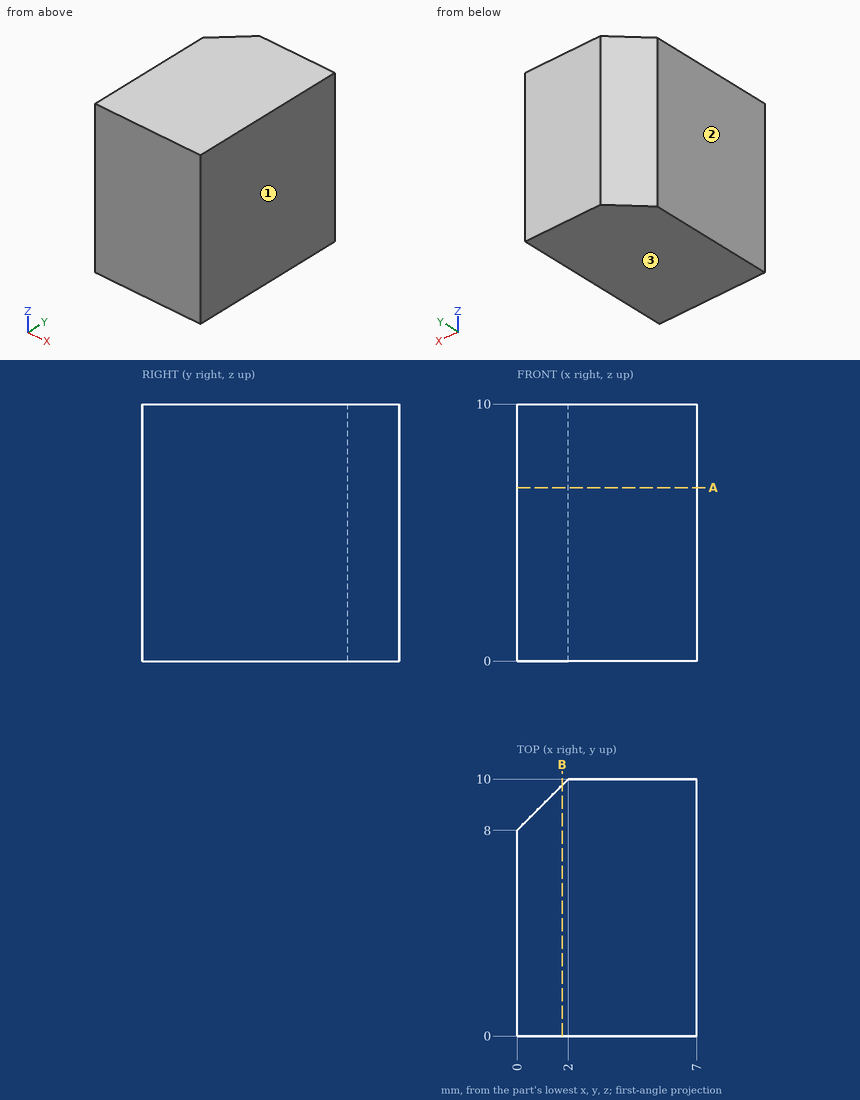
Answer from the drawing. Dimensions are ordinates in mm from the lowest x, y and z of the part. Give positions to 0.01 mm unless a question says otherwise; leave off trailing zeros. Loops run counter-clockwise (first coordinate to the right, second up) from the corner with the lowest first, then second, coordinate; pieces in that order, holes last.
Item 1: Find the intervals of material crossed by line 1 along Y through (x, z) = (0.5, 2.5); line 2 along X through (y, z) = (8.5, 3); line 3 along Y through (x, z) = (1.5, 4.5), in increasing order.
Item 2: The mould has two halves that part along X. Classify the marked faces 1, 2 and 3: released by +X, released by -X, zero draft, split by the parting line, or undercut.
Item 3: The part is cut by section A-A (z = 6.75). Write down the section's boundary in (x, y), and give its area (3 significant figures).
Item 4: The part is cut by section B-B (x = 1.75). Write down the section's boundary in (y, z).
Taken from the geometry:
1. line 1: y = 0 to 8.5
1. line 2: x = 0.5 to 7
1. line 3: y = 0 to 9.5
2. face 1: released by +X
2. face 2: released by -X
2. face 3: zero draft
3. outline: (0, 0) - (7, 0) - (7, 10) - (2, 10) - (0, 8) - close
3. area: 68.0 mm2
4. outline: (0, 0) - (9.75, 0) - (9.75, 10) - (0, 10) - close
